from build123d import *

# Parameters (mm, degrees)
CROQUIS1_W              = 70
CROQUIS1_H              = 80
SALIENTE_EXTRUIR1_DEPTH = 80
CROQUIS2_R              = 30
SALIENTE_EXTRUIR2_DEPTH = 20
CROQUIS3_R              = 21
CORTAR_EXTRUIR1_DEPTH   = 15


with BuildPart() as part:
    # Croquis1 → Saliente-Extruir1 (new body)
    with BuildSketch(Plane.XY):
        with Locations((35, 40)):
            Rectangle(CROQUIS1_W, CROQUIS1_H)
    extrude(amount=SALIENTE_EXTRUIR1_DEPTH)

    # Croquis2 → Saliente-Extruir2 (add)
    with BuildSketch(Plane(origin=(0, 0, 0), x_dir=(-1, 0, 0), z_dir=(0, 0, -1))):
        with Locations((-35, 40)):
            Circle(CROQUIS2_R)
    extrude(amount=SALIENTE_EXTRUIR2_DEPTH)

    # Croquis3 → Cortar-Extruir1 (cut)
    with BuildSketch(Plane.ZY):
        with Locations((40, 40)):
            Circle(CROQUIS3_R)
    extrude(amount=-CORTAR_EXTRUIR1_DEPTH, mode=Mode.SUBTRACT)


solid = part.part
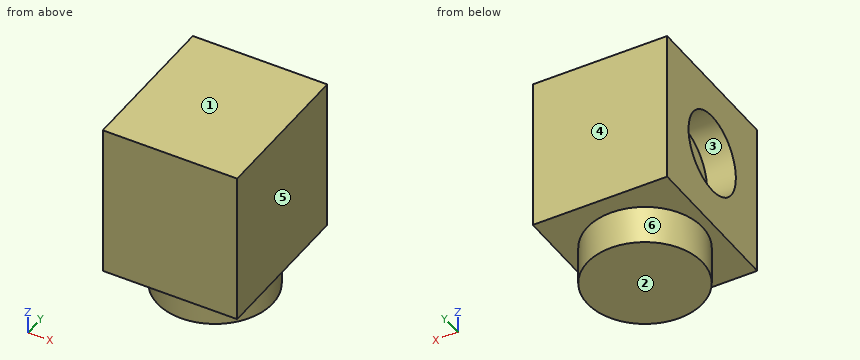
Verification items for the finished model (mm, model axes). Face numbers are marked on the shaded views. A direction names the side the tool comes from. Coordinates: 2 decimals unless noted, no trailing zeros. Write each loop counter-clockwise with the first axis right and the second up, starting at its lowest first coordinate (ties: lowest second). Pieces come first, ordered by that corner, then holes. Notation, with made-up numbers: M -6.75,70 L 11.25,70 A38 cw 11.25,108 Z; hole C -32.5,40.25 d2. An arc over 180 degrees is marked long. Use a Markdown table: item, result.
Q1. Sectioned sample at C-C, the plane z = 59.5. Record the boundary of the cut face in (x, y).
Reply:
| item | result |
|---|---|
| outline | M 0,0 L 70,0 L 70,80 L 0,80 L 0,47.79 L 15,47.79 L 15,32.21 L 0,32.21 Z |
Q2. Thickness scan on line 1 (Y direction, x = 7, z = 40); line 2 (Z direction, x = 11.5, y = 64.5); line 3 (Z direction, x = 7.5, y = 33). Record the ranges inside material, lowest first.
Reply:
| item | result |
|---|---|
| line 1 | y = 0 to 19, 61 to 80 |
| line 2 | z = 0 to 80 |
| line 3 | z = -20 to 20.2, 59.8 to 80 |
Q3. Set-up check for the marked faces 5 and 6: record each of +Z, -Z, +X, -X, +Y, -Y from which the full face is reachable in a straight line by a thin tool's end or side.
Reply:
| item | result |
|---|---|
| face 5 | +Z, -Z, +X, +Y, -Y |
| face 6 | -Z |
Q4. Draft check along Z on the marked faces 1, 2, 3 and 4. Enter one of: +Z half, -Z half, draft (parallel to the pull), parting line (faces both ways), or undercut.
Reply:
| item | result |
|---|---|
| face 1 | +Z half |
| face 2 | -Z half |
| face 3 | undercut |
| face 4 | draft |
Q5. Sectioned sample at B-B, the plane x = 8. Record the boundary of the cut face in (y, z), plus the area to 3 significant figures.
Reply:
| item | result |
|---|---|
| outline | M 0,0 L 26.92,0 L 26.92,-20 L 53.08,-20 L 53.08,0 L 80,0 L 80,80 L 0,80 Z; hole C 40,40 d42 |
| area | 5,540 mm² |
Q6. Sectioned sample at A-A, the plane y = 40. Record the boundary of the cut face in (x, z).
Reply:
| item | result |
|---|---|
| outline | M 0,0 L 5,0 L 5,-20 L 65,-20 L 65,0 L 70,0 L 70,80 L 0,80 L 0,61 L 15,61 L 15,19 L 0,19 Z |
Q7. Sectioned sample at D-D, the plane x = 35. Record the boundary of the cut face in (y, z), plus the area to 3 significant figures.
Reply:
| item | result |
|---|---|
| outline | M 0,0 L 10,0 L 10,-20 L 70,-20 L 70,0 L 80,0 L 80,80 L 0,80 Z |
| area | 7,600 mm² |
